Can you work these out from the model? Positions are in its coordinate system, mm. Face numbers are marked on the shaded views. A direction names the side the tool comes from. Round coordinates to 2 decimals unless told otherwise and drop trailing zeros. Order: outer loops, then holes, each group sorted by start corner. A loop starts at its lowest first (then second) coordinate and runs counter-clockwise, first axis right, second up. Notation, with made-up numbers: M 88,77.5 L 140,77.5 A25 cw 140,98.5 Z; hole C -32,-19 d6. An arc over 180 degrees is marked long. Answer as a JSON object with one key per item and string values. Group by question number.
```python
from build123d import *

# Parameters (mm, degrees)
SKETCH_2_R          = 1.5999999999999899
SKETCH_2_R_2        = 1.6000000000000019
SKETCH_2_R_3        = 1.600000000000012
SKETCH_2_R_4        = 1.5999999999999999
EXTRUDE_1_DEPTH     = 1.5
CUT_EXTRUDE_1_DEPTH = 3
FILLET_1_R          = 1
FILLET_2_R          = 1.75
MOVE_FACE_1_BY      = 0.5
MOVE_FACE_1_2_BY    = 0.5
MOVE_FACE_1_3_BY    = 0.5
MOVE_FACE_1_4_BY    = 0.5
MOVE_FACE_1_5_BY    = 0.5
MOVE_FACE_1_6_BY    = 0.5
MOVE_FACE_1_7_BY    = 0.5
MOVE_FACE_1_8_BY    = 0.5
MOVE_FACE_1_9_BY    = 0.5
MOVE_FACE_1_10_BY   = 0.5
MOVE_FACE_1_11_BY   = 0.5
MOVE_FACE_1_12_BY   = 0.5
MOVE_FACE_1_13_BY   = 0.5
MOVE_FACE_1_14_BY   = 0.5


with BuildPart() as part:
    # ｽｹｯﾁ2 → ﾎﾞｽ - 押し出し1 (new, symmetric)
    with BuildSketch(Plane(origin=(0, 0, 0), x_dir=(1, 0, 0), z_dir=(0, 1, 0))):
        Polygon((24.47000000000005, 8.660254037844277), (9.470000000000297, 1.73e-15), (0, 0), (0, -14.999999999999998), (30.000000000000004, -14.999999999999995), (55.450762113533145, 15.000000000000043), (50.450762113533166, 23.66025403784434), align=None)
        with Locations(Location((48.62063509461097, 16.830127018922173, 0), (0, 0, 270))):
            Circle(SKETCH_2_R, mode=Mode.SUBTRACT)
        with Locations(Location((25, -7.5, 0), (0, 0, 270))):
            Circle(SKETCH_2_R_2, mode=Mode.SUBTRACT)
        with Locations(Location((31.300127018922208, 6.830127018922147, 0), (0, 0, 270))):
            Circle(SKETCH_2_R_3, mode=Mode.SUBTRACT)
        with Locations(Location((5, -7.5, 0), (0, 0, 270))):
            Circle(SKETCH_2_R_4, mode=Mode.SUBTRACT)
    extrude(amount=EXTRUDE_1_DEPTH, both=True)

    # ｽｹｯﾁ3 → ｶｯﾄ - 押し出し1 (cut)
    with BuildSketch(Plane(origin=(0, 1.5, 0), x_dir=(1, 0, 0), z_dir=(0, 1, 0))):
        Polygon((26.470000000000045, 5.196152422706529), (17.470000000000258, -3.55e-15), (27.140628594077313, 0), (27.879009742330265, 2.755675960631065), align=None)
        Polygon((33.35228567653781, 0), (37.47986861759486, 0), (45.16947255557436, 9.064094706096034), (34.06279326771847, 2.651650429449568), align=None)
        Polygon((31.446764780347493, -7.111500799466448), (37.47986861759486, 3.55e-15), (33.35228567653781, 0), align=None)
    extrude(amount=-CUT_EXTRUDE_1_DEPTH, mode=Mode.SUBTRACT)

    # ﾌｨﾚｯﾄ1
    fillet_1_edges = [part.edges().sort_by_distance(p)[0] for p in [
        (27.87900974233027, 0, -2.7556759606310655),
        (27.140628594077313, 0, -8.9e-16),
        (17.47000000000026, 0, 1.78e-15),
        (26.47000000000005, 0, -5.19615242270653),
        (34.06279326771847, 0, -2.6516504294495666),
        (45.16947255557436, 0, -9.064094706096032),
        (31.446764780347493, 0, 7.111500799466448),
    ]]
    fillet(fillet_1_edges, radius=FILLET_1_R)

    # ﾌｨﾚｯﾄ2
    fillet_2_edges = [part.edges().sort_by_distance(p)[0] for p in [
        (50.450762113533166, 0, -23.66025403784434),
        (55.450762113533145, 0, -15.000000000000043),
        (30.000000000000004, 0, 14.999999999999995),
        (0, 0, 14.999999999999998),
        (0, 0, 0),
        (9.470000000000297, 0, -1.73e-15),
    ]]
    fillet(fillet_2_edges, radius=FILLET_2_R)

    # Move Face 1: a face moved inward by 0.5
    extrude(part.faces().sort_by_distance((33.277523818, 0, 0.279015055))[0], amount=MOVE_FACE_1_BY, dir=(-0.965925826, 0, -0.258819045), mode=Mode.SUBTRACT)

    # Move Face 1 2: a curved face moved inward by 0.5
    add(Solid.thicken(part.faces().sort_by_distance((33.10124082, 0, 3.954158856))[0], -MOVE_FACE_1_2_BY), mode=Mode.SUBTRACT)

    # Move Face 1 3: a face moved inward by 0.5
    extrude(part.faces().sort_by_distance((37.884808697, 0, -0.477321752))[0], amount=MOVE_FACE_1_3_BY, dir=(0.762556575, 0, 0.646921533), mode=Mode.SUBTRACT)

    # Move Face 1 4: a curved face moved inward by 0.5
    add(Solid.thicken(part.faces().sort_by_distance((41.44689767, 0, -5.957600166))[0], -MOVE_FACE_1_4_BY), mode=Mode.SUBTRACT)

    # Move Face 1 5: a face moved inward by 0.5
    extrude(part.faces().sort_by_distance((37.300315213, 0, -4.520834596))[0], amount=MOVE_FACE_1_5_BY, dir=(-0.5, 0, -0.866025404), mode=Mode.SUBTRACT)

    # Move Face 1 6: a curved face moved inward by 0.5
    add(Solid.thicken(part.faces().sort_by_distance((34.128159395, 0, -2.601493236))[0], -MOVE_FACE_1_6_BY), mode=Mode.SUBTRACT)

    # Move Face 1 7: a curved face moved inward by 0.5
    add(Solid.thicken(part.faces().sort_by_distance((20.236124981, 0, -0.741180955))[0], -MOVE_FACE_1_7_BY), mode=Mode.SUBTRACT)

    # Move Face 1 8: a face moved inward by 0.5
    extrude(part.faces().sort_by_distance((23.787676207, 0, 0))[0], amount=MOVE_FACE_1_8_BY, dir=(0, 0, 1), mode=Mode.SUBTRACT)

    # Move Face 1 9: a curved face moved inward by 0.5
    add(Solid.thicken(part.faces().sort_by_distance((26.982063035, 0, -0.20664666))[0], -MOVE_FACE_1_9_BY), mode=Mode.SUBTRACT)

    # Move Face 1 10: a face moved inward by 0.5
    extrude(part.faces().sort_by_distance((27.555515408, 0, -1.548378669))[0], amount=MOVE_FACE_1_10_BY, dir=(0.965925826, 0, 0.258819045), mode=Mode.SUBTRACT)

    # Move Face 1 11: a curved face moved inward by 0.5
    add(Solid.thicken(part.faces().sort_by_distance((27.797322419, 0, -2.74492162))[0], -MOVE_FACE_1_11_BY), mode=Mode.SUBTRACT)

    # Move Face 1 12: a face moved inward by 0.5
    extrude(part.faces().sort_by_distance((27.320951481, 0, -3.722261224))[0], amount=MOVE_FACE_1_12_BY, dir=(0.866025404, 0, -0.5), mode=Mode.SUBTRACT)

    # Move Face 1 13: a curved face moved inward by 0.5
    add(Solid.thicken(part.faces().sort_by_distance((26.362793641, 0, -4.796052845))[0], -MOVE_FACE_1_13_BY), mode=Mode.SUBTRACT)

    # Move Face 1 14: a face moved inward by 0.5
    extrude(part.faces().sort_by_distance((23.153012702, 0, -3.281088913))[0], amount=MOVE_FACE_1_14_BY, dir=(-0.5, 0, -0.866025404), mode=Mode.SUBTRACT)


solid = part.part
```
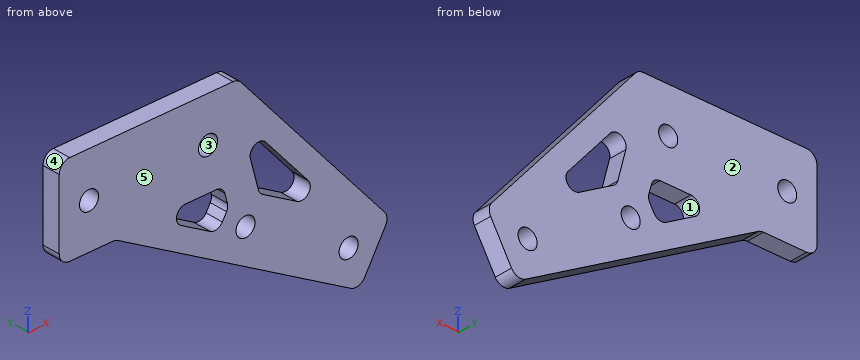
1) If we section it at D-D on z = 7.5: Write out the boundary of the cut face in (x, y), plus the area to 3 significant figures.
2) Which directions (+Z, -Z, +X, -X, +Y, -Y) give clear straight access to the entire face, cutting with the end or side of a thin tool? Please do the marked faces 1 and 2.
3) If we section it at A-A on x = 5: Write out the boundary of the cut face in (y, z), plus the area to 3 significant figures.
4) If we section it at C-C on y = 0.85: Count the separate pieces of the cut face and the enclosed holes in it, plus the area to 3 significant figures.
5) I need wall thicknesses on line 1 along X through (y, z) = (0, 7.5); line 2 along X through (y, z) = (1.35, -3); line 3 along Z through (x, y) = (21.5, 0.95). Which ranges of each line are inside material? Lowest first, please.
6) For pin 1 (2.5 mm diameter, centred on x = 31.3, z = -6.83, fed in from -Y); pin 2 (0.9 mm diameter, centred on x = 5.5, y = 0.5, fed in from -Z); pin 3 (1.5 mm diameter, centred on y = -0.5, z = -0.5, fed in from +X); pin 4 (1.5 mm diameter, centred on x = 34, y = -1, fed in from +Z), each with a flat end and sliding along its axis, tell me the tip position at first contact or that it passes through.
7) If we section it at B-B on z = -7.5: Write out the boundary of the cut face in (x, y), plus the area to 3 significant figures.
8) We'd pull the mould along Z, two halves only. Please class the marked faces 3, 4 and 5: +Z half, -Z half, draft (parallel to the pull), parting line (faces both ways), or undercut.
Findings:
{
 "1": {"outline": "M 0,-1.5 L 3.4,-1.5 L 3.4,1.5 L 0,1.5 Z; M 6.6,-1.5 L 23.4,-1.5 L 23.4,1.5 L 6.6,1.5 Z; M 26.6,-1.5 L 36.36,-1.5 L 36.36,1.5 L 26.6,1.5 Z", "area": "89.9 mm^2"},
 "2": {"face 1": "+Y, -Y", "face 2": "+Z, -Z, +X, -X, +Y"},
 "3": {"outline": "M -1.5,0 L 1.5,0 L 1.5,5.9 L -1.5,5.9 Z; M -1.5,9.1 L 1.5,9.1 L 1.5,15 L -1.5,15 Z", "area": "35.4 mm^2"},
 "4": {"separate pieces": "1", "enclosed holes": "6", "area": "907 mm^2"},
 "5": {"line 1": "x = 0 to 3.4, 6.6 to 23.4, 26.6 to 36.36", "line 2": "x = 14.67 to 21.67, 28.26 to 33.81, 40.68 to 45.27", "line 3": "z = -6.95 to -2.9, 0.5 to 15"},
 "6": {"pin 1": "passes through", "pin 2": "stops at z = 0", "pin 3": "stops at x = 43.79", "pin 4": "stops at z = 11.17"},
 "7": {"outline": "M 22.46,-1.5 L 29.85,-1.5 L 29.85,1.5 L 22.46,1.5 Z; M 32.75,-1.5 L 49.09,-1.5 L 49.09,1.5 L 32.75,1.5 Z", "area": "71.2 mm^2"},
 "8": {"face 3": "undercut", "face 4": "+Z half", "face 5": "draft"}
}
